Geometry check sheet. Reference: the model listing, model coordinates, mm. A direction names the side the tool comes from. Round coordinates to 2 decimals unless told otherwise and drop trailing zeros. Order: outer loops, then holes, each group sorted by start corner. A loop starts at its lowest first (then second) coordinate and runs counter-clockwise, first axis right, second up. Notation, with made-up numbers: (3.25, 83) - (58.25, 83) arc R25 cw to (58.25, 115) - close; hole circle Ø10 at (11, 36.25). An arc over 180 degrees is marked (long way). Return JSON: item names as keys, results as strings. Group by question number.
Q1. Gauge pin test, flat ends, axial feed: pin 1 Ø8 at (y, z) = (-12, -2) entering from -X; pin 2 Ø10.5 at (x, y) = (-1.5, 4) entering from +Z; pin 3 Ø4 at (x, y) = (-14.5, 4.5) entering from +Z; pin 4 Ø19 at (x, y) = (5, 0) entering from +Z. Record the tip position at first contact, or that the pin passes through.
Q2. Draft check along Y on faces 1 (the conical face through (6.606, 12.702, -5.508)), 2 (the flat face through (-11.2, -0.1, -12.7)), 3 (the flat face through (12.4, 4, -12.7)), 4 (the flat face through (4, 5, 7.287)). Enter one of: pulls with the +Y half, pulls with the -Y half, needs draft (parallel to the pull), parting line crosses it, or undercut.
Q3. Material ranges on line 1 along Y through (x, z) = (0, -10.25); line 2 along Y through (x, z) = (-2.5, -17.5); line 3 along Y through (x, z) = (-7, 5), recorded low to high.
Q4. Sectioned sample at A-A, the plane z = 10. Record the cut outline in (x, y).
Q5. Sectioned sample at C-C, the plane z = -9. Record the cut outline in (x, y), then the cut area to 3 significant figures.
Q6. Tool access check on faces 5 (the conical face through (6.606, 12.702, -7.192)), 6 (the cylindrical face through (-2.75, -12.4, 6.26)), 7 (the flat face through (4, 5, -19.987)). Record the directions out of +Z, -Z, +X, -X, +Y, -Y that give a thin tool (end or side, any length) a straight path to the whole face; none if there is none.
```python
from build123d import *
from build123d.topology import SkipClean

# Parameters (mm, degrees)
SKETCH1_R           = 12.7
SKETCH1_R_2         = 11
BOSS_EXTRUDE1_DEPTH = 12.7


with BuildPart() as part:
    # Sketch1 → Boss-Extrude1 (new body)
    with BuildSketch(Plane.XY):
        Circle(SKETCH1_R)
        with Locations((-0.762, 0)):
            Circle(SKETCH1_R_2, mode=Mode.SUBTRACT)
    extrude(amount=BOSS_EXTRUDE1_DEPTH)

    # Sketch2 → Revolve1 (revolve)
    with BuildSketch(Plane(origin=(0, 0, 0), x_dir=(0, 0, -1), z_dir=(1, 0, 0)), mode=Mode.PRIVATE) as revolve1_sk:
        with BuildLine():
            Line((-7.2874886, 11), (-7.2874886, 6))
            Line((-7.2874886, 6), (6.35, 6))
            Line((6.35, 6), (6.35, 13.62))
            ThreePointArc((6.35, 13.62), (5.969, 13.722088642), (5.690088642, 14.001))
            Line((5.690088642, 14.001), (2.775047133, 19.05))
            Line((2.775047133, 19.05), (0, 19.05))
            Line((0, 19.05), (0, 11))
            Line((0, 11), (-7.2874886, 11))
        make_face()
    revolve(revolve1_sk.sketch.rotate(Axis((0, 0, 0), (0, 0, -1)), 90), axis=Axis((0, 0, 0), (0, 0, -1)))

    # Mirror1: part across plane


with BuildPart() as part_1:
    with SkipClean():  # the faces are left unmerged after this step: merging them gives an invalid solid
        add(part.part)
        add(part.part.mirror(Plane(origin=(0, 6, -6.35), x_dir=(1, 0, 0), z_dir=(0, 0, 1))))


solid = part_1.part
```
Reply:
{
 "1": {"pin 1": "x = -17.29", "pin 2": "z = 7.29", "pin 3": "z = 0", "pin 4": "z = 12.7"},
 "2": {"face 1": "parting line crosses it", "face 2": "undercut", "face 3": "needs draft", "face 4": "undercut"},
 "3": {"line 1": "-19.05 to -6, 6 to 19.05", "line 2": "-12.45 to -10.86, -10.71 to -5.45, 5.45 to 10.71, 10.86 to 12.45", "line 3": "-10.6 to -9.06, -8.49 to 8.49, 9.06 to 10.6"},
 "4": {"outline": "circle Ø25.4 at (0, 0); hole circle Ø22 at (-0.76, 0)"},
 "5": {"outline": "circle Ø34.9 at (0, 0); hole circle Ø12 at (0, 0)", "area": "843 mm^2"},
 "6": {"face 5": "none", "face 6": "+Z", "face 7": "-Z"}
}
